```python
from build123d import *

# Parameters (mm, degrees)
SKETCH1_W           = 50
SKETCH1_H           = 50
SKETCH1_R           = 3
BOSS_EXTRUDE1_DEPTH = 3
SKETCH2_R           = 5.3
CUT_EXTRUDE1_DEPTH  = 1.5


with BuildPart() as part:
    # Sketch1 → Boss-Extrude1 (new body)
    with BuildSketch(Plane(origin=(0, 0, 0), x_dir=(1, 0, 0), z_dir=(0, 1, 0))):
        Rectangle(SKETCH1_W, SKETCH1_H)
        with Locations(Location((-17.5, 17.5, 0), (0, 0, 270))):
            Circle(SKETCH1_R, mode=Mode.SUBTRACT)
        with Locations(Location((17.5, 17.5, 0), (0, 0, 270))):
            Circle(SKETCH1_R, mode=Mode.SUBTRACT)
        with Locations(Location((-17.5, -17.5, 0), (0, 0, 270))):
            Circle(SKETCH1_R, mode=Mode.SUBTRACT)
        with Locations(Location((17.5, -17.5, 0), (0, 0, 270))):
            Circle(SKETCH1_R, mode=Mode.SUBTRACT)
    extrude(amount=BOSS_EXTRUDE1_DEPTH)

    # Sketch2 → Cut-Extrude1 (cut)
    with BuildSketch(Plane(origin=(0, 3, 0), x_dir=(1, 0, 0), z_dir=(0, 1, 0))):
        with Locations(Location((-17.5, 17.5, 0), (0, 0, 270))):
            Circle(SKETCH2_R)
        with Locations(Location((17.5, 17.5, 0), (0, 0, 270))):
            Circle(SKETCH2_R)
        with Locations(Location((17.5, -17.5, 0), (0, 0, 270))):
            Circle(SKETCH2_R)
        with Locations(Location((-17.5, -17.5, 0), (0, 0, 270))):
            Circle(SKETCH2_R)
    extrude(amount=-CUT_EXTRUDE1_DEPTH, mode=Mode.SUBTRACT)


solid = part.part
```
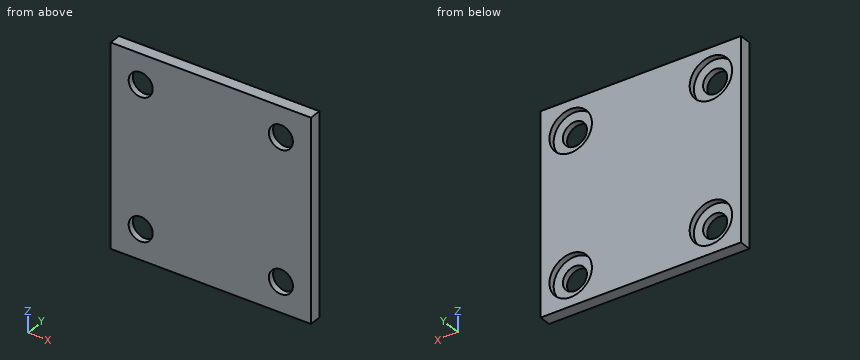
Source: CAD feature listing. Evaluate the final solid. Frame: model axes, mm. Round coordinates to 2 decimals unless told otherwise and drop trailing zeros. Write each loop counter-clockwise with the first axis right and the second up, starting at its lowest first coordinate (ties: lowest second). Pieces come first, ordered by that corner, then holes. Notation, with made-up numbers: M -0.75,65 L 47.25,65 A29 cw 47.25,86 Z; hole C 47.5,52.5 d11. An arc over 180 degrees is marked long. Use CSV: the item, a comma, the result in double quotes. Start each with the question number.
Q1. Cut plane C-C on y = 0.45. Output: boundary loops of the cut face in (x, z).
Q2. Line query: line 1 (X direction, y = 0.6, z = -17.5); line 2 (X direction, y = 2.05, z = 17.5). Output: solid intervals per line, ascending. Write a range as from..to.
Q3. First-contact query: P1, Ø8.5, axis at x = -17.5, z = -17.5, coming from the +Y side; P2, Ø5, axis at x = 17.5, z = 17.5, coming from the +Y side; P3, Ø11.5, axis at x = -17, z = 15, coming from the +Y side. Flat tips, straight axial feed; report the tip coordinate or a pass-through.
Q4. Cut plane B-B on x = -17.5. Output: boundary loops of the cut face in (y, z), plus the area to 3 significant figures.
Q5. Cut plane A-A on z = 17.5. Output: boundary loops of the cut face in (x, y), plus the area to 3 significant figures.
Results found:
1,outline,"M -25,-25 L 25,-25 L 25,25 L -25,25 Z; hole C -17.5,-17.5 d6; hole C -17.5,17.5 d6; hole C 17.5,-17.5 d6; hole C 17.5,17.5 d6"
2,line 1,"-25..-20.5, -14.5..14.5, 20.5..25"
2,line 2,"-25..-22.8, -12.2..12.2, 22.8..25"
3,P1,"y = 1.5"
3,P2,"through"
3,P3,"y = 3"
4,outline,"M 0,-25 L 3,-25 L 3,-22.8 L 1.5,-22.8 L 1.5,-20.5 L 0,-20.5 Z; M 0,-14.5 L 1.5,-14.5 L 1.5,-12.2 L 3,-12.2 L 3,12.2 L 1.5,12.2 L 1.5,14.5 L 0,14.5 Z; M 0,20.5 L 1.5,20.5 L 1.5,22.8 L 3,22.8 L 3,25 L 0,25 Z"
4,area,"100 mm^2"
5,outline,"M -25,0 L -20.5,0 L -20.5,1.5 L -22.8,1.5 L -22.8,3 L -25,3 Z; M -14.5,0 L 14.5,0 L 14.5,1.5 L 12.2,1.5 L 12.2,3 L -12.2,3 L -12.2,1.5 L -14.5,1.5 Z; M 20.5,0 L 25,0 L 25,3 L 22.8,3 L 22.8,1.5 L 20.5,1.5 Z"
5,area,"100 mm^2"
